from build123d import *

# Parameters (mm, degrees)
SKETCH1_W                                = 75.85
SKETCH1_H                                = 10
M3_5_CLEARANCE_HOLE1_D                   = 4.1656
M3_5_CLEARANCE_HOLE1_DEPTH               = 10
M3_CLEARANCE_HOLE1_D                     = 3.4544
M3_CLEARANCE_HOLE1_DEPTH                 = 10
F_12_5_12_5_DIAMETER_HOLE1_D             = 12.5
F_12_5_12_5_DIAMETER_HOLE1_DEPTH         = 10
CBORE_FOR_M90_HEX_HEAD_BOLT1_D           = 97.8
CBORE_FOR_M90_HEX_HEAD_BOLT1_DEPTH       = 10
CBORE_FOR_M90_HEX_HEAD_BOLT1_CBORE_D     = 101.8
CBORE_FOR_M90_HEX_HEAD_BOLT1_CBORE_DEPTH = 7


with BuildPart() as part:
    # Sketch1 → Revolve1 (revolve)
    with BuildSketch(Plane.XZ):
        with Locations((37.925, 0)):
            Rectangle(SKETCH1_W, SKETCH1_H)
    revolve(axis=Axis((0, 0, 5), (0, 0, -1)))

    # M3.5 Clearance Hole1
    with Locations(Plane(origin=(0, 0, -5), x_dir=(-1, 0, 0), z_dir=(0, 0, -1))):
        with Locations((60.051933549, 34.671), (-34.671, 60.051933549), (-60.051933549, -34.671), (34.671, -60.051933549)):
            Hole(M3_5_CLEARANCE_HOLE1_D / 2, depth=M3_5_CLEARANCE_HOLE1_DEPTH)

    # M3 Clearance Hole1
    with Locations(Plane(origin=(0, 0, -5), x_dir=(-1, 0, 0), z_dir=(0, 0, -1))):
        with Locations((41.931432124, 41.931432124), (57.279401499, 15.347969375), (57.279401499, -15.347969375), (41.931432124, -41.931432124), (15.347969375, -57.279401499), (-15.347969375, -57.279401499), (-41.931432124, -41.931432124), (-57.279401499, -15.347969375), (-57.279401499, 15.347969375), (-41.931432124, 41.931432124), (-15.347969375, 57.279401499), (15.347969375, 57.279401499)):
            Hole(M3_CLEARANCE_HOLE1_D / 2, depth=M3_CLEARANCE_HOLE1_DEPTH)

    # Ø12.5 (12.5) Diameter Hole1
    with Locations(Plane(origin=(0, 0, -5), x_dir=(-1, 0, 0), z_dir=(0, 0, -1))):
        with Locations((62.85, 0), (0, -62.85), (-62.85, 0), (0, 62.85)):
            Hole(F_12_5_12_5_DIAMETER_HOLE1_D / 2, depth=F_12_5_12_5_DIAMETER_HOLE1_DEPTH)

    # CBORE for M90 Hex Head Bolt1
    with Locations(Plane.XY.offset(5)):
        with Locations((0, 0)):
            CounterBoreHole(CBORE_FOR_M90_HEX_HEAD_BOLT1_D / 2, CBORE_FOR_M90_HEX_HEAD_BOLT1_CBORE_D / 2, CBORE_FOR_M90_HEX_HEAD_BOLT1_CBORE_DEPTH, depth=CBORE_FOR_M90_HEX_HEAD_BOLT1_DEPTH)


solid = part.part
Model file for the job. Use its own axes, mm. Coordinates: 2 decimals unless noted, no trailing zeros. Order: outer loops, then holes, each group sorted by start corner. A loop starts at its lowest first (then second) coordinate and runs counter-clockwise, first axis right, second up. Notation, with made-up numbers: (5, -26) -> (56, -26) arc R26 ccw to (56, 13) -> close; hole circle Ø6 at (30, -7.5). An arc over 180 degrees is marked (long way). Return JSON: item names as keys, results as strings. Group by question number.
Item 1: Pull direction X, two halves, no side cores. Call faces 1 (the flat face through (1, 50, -5)), 2 (the cylindrical face through (-16.443, 74.046, 0.07)), 3 (the cylindrical face through (27.36, 42.92, 1.55)): pulls with the +X half, pulls with the -X half, needs draft (parallel to the pull), parting line crosses it, or undercut.
Item 2: Saw through at A-A on y = 0. Write the cut outline in (x, z).
Item 3: Wall check: line 1 along Y through (x, z) = (0, 3); line 2 along Y through (x, z) = (15, 0.25); line 3 along Y through (x, z) = (-36.5, -0.5). Give the ranges that are in metal, low to high. Write a range as [from, to].
Item 4: Saw through at D-D on x = 30. Write the cut outline in (y, z), then the cut area to 3 significant figures.
Item 5: Flat gauge pins, fed straight in: P1, Ø1, axis at x = 46, z = 3, coming from the -Y side; P2, Ø3, axis at x = 13.5, z = 0, coming from the +Y side; P3, Ø3, axis at x = -25, z = 0.5, coming from the -Y side. Where does each tip first touch, or does it go through?
Item 6: Saw through at C-C on z = -3.5. State how many separate pieces and enclosed holes the cut face has, then the cut area to 3 significant figures.
Values found:
{
 "1": {"face 1": "needs draft", "face 2": "parting line crosses it", "face 3": "undercut"},
 "2": {"outline": "(-75.85, -5) -> (-69.1, -5) -> (-69.1, 5) -> (-75.85, 5) -> close; (-56.6, -5) -> (-48.9, -5) -> (-48.9, -2) -> (-50.9, -2) -> (-50.9, 5) -> (-56.6, 5) -> close; (48.9, -5) -> (56.6, -5) -> (56.6, 5) -> (50.9, 5) -> (50.9, -2) -> (48.9, -2) -> close; (69.1, -5) -> (75.85, -5) -> (75.85, 5) -> (69.1, 5) -> close"},
 "3": {"line 1": "y = [-75.85, -69.1], [-56.6, -50.9], [50.9, 56.6], [69.1, 75.85]", "line 2": "y = [-74.35, -58.97], [-55.59, -48.64], [48.64, 55.59], [58.97, 74.35]", "line 3": "y = [-66.49, -61.05], [-59.06, -35.48], [35.48, 66.49]"},
 "4": {"outline": "(-69.67, -5) -> (-38.62, -5) -> (-38.62, -2) -> (-41.12, -2) -> (-41.12, 5) -> (-69.67, 5) -> close; (38.62, -5) -> (69.67, -5) -> (69.67, 5) -> (41.12, 5) -> (41.12, -2) -> (38.62, -2) -> close", "area": "586 mm2"},
 "5": {"P1": "stops at y = -60.69", "P2": "stops at y = 74.89", "P3": "stops at y = -72.12"},
 "6": {"separate pieces": "1", "enclosed holes": "21", "area": "9,900 mm2"}
}
